Could you check a few things on this drawing? It's one solid part, dimensions in mm from its lowest x, y, z. Coordinates: 2 decimals unless noted, no trailing zeros. Loops run counter-clockwise (first coordinate to the right, second up) from the corner with the lowest first, then second, coordinate; pieces in that order, holes last.
1) Imagine slicing it at A-A on z = 6.5. Please give me the cut outline in (x, y), plus the area to 3 significant figures.
2) Thinking about a two-plate mould opening in Z: for the marked faces 1, 2 and 3, which applies, released by +Z, released by -Z, zero draft, split by the parting line, or undercut?
3) Imagine slicing it at C-C on z = 10.75. Please give me the cut outline in (x, y), plus the area to 3 significant figures.
4) Imagine slicing it at B-B on x = 6.5. Please give me the cut outline in (y, z), plus the area to 3 significant figures.
5) If I drill on line 1 along Z through (x, y) = (6.5, 5.25); line 2 along Y through (x, z) = (2.25, 8.5); line 3 along Z through (x, y) = (8, 14), over which ranges is the centre line in solid material (lowest first)?
6) Imagine slicing it at D-D on y = 8.25. Please give me the cut outline in (x, z).
7) Will these pins go through, and if not, where does the flat tip stop? P1, Ø4, axis at x = 11, y = 5.5, coming from the -Z side; P2, Ø1.5, axis at y = 7, z = 11.5, coming from the +X side; P3, Ø4, axis at x = 9.5, z = 5.5, coming from the -Y side.
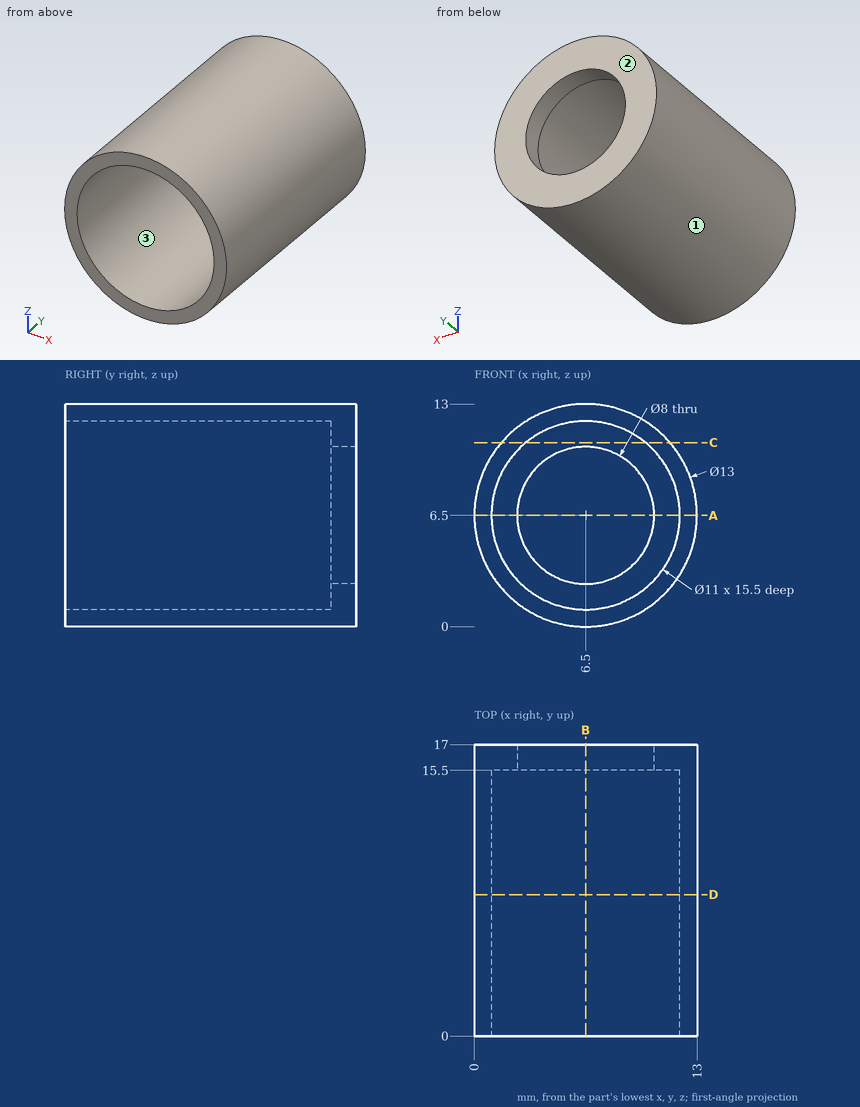
Filled in:
1. outline: (0, 0) - (1, 0) - (1, 15.5) - (2.5, 15.5) - (2.5, 17) - (0, 17) - close; (10.5, 15.5) - (12, 15.5) - (12, 0) - (13, 0) - (13, 17) - (10.5, 17) - close
1. area: 38.5 mm2
2. face 1: split by the parting line
2. face 2: zero draft
2. face 3: undercut
3. outline: (1.58, 0) - (3.01, 0) - (3.01, 15.5) - (9.99, 15.5) - (9.99, 0) - (11.42, 0) - (11.42, 17) - (1.58, 17) - close
3. area: 59.0 mm2
4. outline: (0, 0) - (17, 0) - (17, 2.5) - (15.5, 2.5) - (15.5, 1) - (0, 1) - close; (0, 12) - (15.5, 12) - (15.5, 10.5) - (17, 10.5) - (17, 13) - (0, 13) - close
4. area: 38.5 mm2
5. line 1: z = 0 to 1, 12 to 13
5. line 2: y = 15.5 to 17
5. line 3: z = 0.18 to 1.21, 11.79 to 12.82
6. outline: circle Ø13 at (6.5, 6.5); hole circle Ø11 at (6.5, 6.5)
7. P1: stops at z = 0.5
7. P2: stops at x = 11.42
7. P3: stops at y = 15.5
